```python
from build123d import *

# Parameters (mm, degrees)
SKETCH_2_W                   = 62
SKETCH_2_H                   = 45
EXTRUDE_3_DEPTH              = 8
SKETCH_3_W                   = 3.004963504
SKETCH_3_H                   = 5
CUT_EXTRUDE_1_DEPTH          = 58.648048048
EXTRUDE_4_DEPTH              = 3
SKETCH_6_W                   = 3
SKETCH_6_H                   = 5
EXTRUDE_5_DEPTH              = 2
SKETCH_7_W                   = 3
SKETCH_7_H                   = 5
EXTRUDE_6_DEPTH              = 2
SKETCH_8_W                   = 49.990072992
SKETCH_8_H                   = 5
EXTRUDE_7_DEPTH              = 2
SKETCH_9_W                   = 3
SKETCH_9_H                   = 5
CUT_EXTRUDE_2_DEPTH          = 66.65020057
SKETCH_10_W                  = 3
SKETCH_10_H                  = 5
CUT_EXTRUDE_4_DEPTH          = 66.65020057
SKETCH_11_W                  = 49.990072992
SKETCH_11_H                  = 5
EXTRUDE_8_DEPTH              = 17
SKETCH_12_W                  = 49.990072992
SKETCH_12_H                  = 3
EXTRUDE_9_DEPTH              = 25
EXTRUDE_START                = 3.72
SKETCH_16_W                  = 49.990072992
SKETCH_16_H                  = 25
EXTRUDE_10_DEPTH             = 3
SKETCH_17_W                  = 49.990072992
SKETCH_17_H                  = 25
CUT_EXTRUDE_5_DEPTH          = 81.043408441
SKETCH_18_W                  = 84
SKETCH_18_H                  = 3
EXTRUDE_11_DEPTH             = 20
HOLE_WIZARD_M3_2_D           = 2.5
HOLE_WIZARD_M3_2_CSINK_D     = 3.05
HOLE_WIZARD_M3_2_CSINK_ANGLE = 90


with BuildPart() as part:
    # 草图2 → 凸台-拉伸3 (new body)
    with BuildSketch(Plane.XY):
        with Locations((-4.132569558, -3.93531014)):
            Rectangle(SKETCH_2_W, SKETCH_2_H)
    extrude(amount=EXTRUDE_3_DEPTH)

    # 草图3 → 切除-拉伸1 (cut, through all)
    with BuildSketch(Plane.XZ.offset(26.43531014)):
        with Locations((-30.630087806, 5.5)):
            Rectangle(SKETCH_3_W, SKETCH_3_H)
        with Locations((22.36494869, 5.5)):
            Rectangle(SKETCH_3_W, SKETCH_3_H)
    extrude(amount=-CUT_EXTRUDE_1_DEPTH, mode=Mode.SUBTRACT)

    # 草图5 → 凸台-拉伸4 (add)
    with BuildSketch(Plane(origin=(0, 0, 0), x_dir=(-1, 0, 0), z_dir=(0, 0, -1))):
        Polygon((-38.867430442, -45.43531014), (-38.867430442, 18.56468986), (45.132569558, 18.56468986), (45.132569558, -45.43531014), (3.132569558, -45.43531014), align=None)
    extrude(amount=-EXTRUDE_4_DEPTH)

    # 草图6 → 凸台-拉伸5 (add)
    with BuildSketch(Plane.XZ.offset(26.43531014)):
        with Locations((-33.632569558, 5.5)):
            Rectangle(SKETCH_6_W, SKETCH_6_H)
    extrude(amount=EXTRUDE_5_DEPTH)

    # 草图7 → 凸台-拉伸6 (add)
    with BuildSketch(Plane.XZ.offset(26.43531014)):
        with Locations((25.367430442, 5.5)):
            Rectangle(SKETCH_7_W, SKETCH_7_H)
    extrude(amount=EXTRUDE_6_DEPTH)

    # 草图8 → 凸台-拉伸7 (add)
    with BuildSketch(Plane.XZ.offset(26.43531014)):
        with Locations((-4.132569558, 5.5)):
            Rectangle(SKETCH_8_W, SKETCH_8_H)
    extrude(amount=EXTRUDE_7_DEPTH)

    # 草图9 → 切除-拉伸2 (cut, through all)
    with BuildSketch(Plane.XZ.offset(28.43531014)):
        with Locations((-33.632569558, 5.5)):
            Rectangle(SKETCH_9_W, SKETCH_9_H)
    extrude(amount=-CUT_EXTRUDE_2_DEPTH, mode=Mode.SUBTRACT)

    # 草图10 → 切除-拉伸4 (cut, through all)
    with BuildSketch(Plane.XZ.offset(28.43531014)):
        with Locations((25.367430442, 5.5)):
            Rectangle(SKETCH_10_W, SKETCH_10_H)
    extrude(amount=-CUT_EXTRUDE_4_DEPTH, mode=Mode.SUBTRACT)

    # 草图11 → 凸台-拉伸8 (add)
    with BuildSketch(Plane.XZ.offset(28.43531014)):
        with Locations((-4.132569558, 5.5)):
            Rectangle(SKETCH_11_W, SKETCH_11_H)
    extrude(amount=EXTRUDE_8_DEPTH)

    # 草图12 → 凸台-拉伸9 (add)
    with BuildSketch(Plane.XY.offset(8)):
        with Locations((-4.132569558, -43.93531014)):
            Rectangle(SKETCH_12_W, SKETCH_12_H)
    extrude(amount=EXTRUDE_9_DEPTH)

    # 草图16 → 凸台-拉伸10 (add)
    with BuildSketch(Plane(origin=(0, -42.43531014, 0), x_dir=(1, 0, 0), z_dir=(0, 1, 0)).offset(EXTRUDE_START)):
        with Locations((-4.132569558, -20.5)):
            Rectangle(SKETCH_16_W, SKETCH_16_H)
    extrude(amount=EXTRUDE_10_DEPTH)

    # 草图17 → 切除-拉伸5 (cut, through all)
    with BuildSketch(Plane.XZ.offset(38.71531014)):
        with Locations((-4.132569558, 20.5)):
            Rectangle(SKETCH_17_W, SKETCH_17_H)
    extrude(amount=CUT_EXTRUDE_5_DEPTH, mode=Mode.SUBTRACT)

    # 草图18 → 凸台-拉伸11 (add)
    with BuildSketch(Plane.XZ.offset(45.43531014)):
        with Locations((-3.132569558, 1.5)):
            Rectangle(SKETCH_18_W, SKETCH_18_H)
    extrude(amount=EXTRUDE_11_DEPTH)

    # M3 螺纹孔2 (through all)
    with Locations(Plane.XY.offset(3)):
        with Locations((-43.132569558, -3.43531014), (36.867430442, -3.43531014), (36.867430442, -63.43531014), (-43.132569558, -63.43531014)):
            CounterSinkHole(HOLE_WIZARD_M3_2_D / 2, HOLE_WIZARD_M3_2_CSINK_D / 2, counter_sink_angle=HOLE_WIZARD_M3_2_CSINK_ANGLE)


solid = part.part
```
The listing builds one solid part. Answer for the finished solid, in the listing's coordinates (mm). A direction names the side the tool comes from. Give positions to 0.01 mm unless a question says otherwise; leave off trailing zeros. Write each loop counter-clockwise with the first axis right and the second up, starting at its lowest first coordinate (ties: lowest second). Pieces come first, ordered by that corner, then holes. Notation, with made-up numbers: (16.25, 86) -> (41.25, 86) arc R26 ccw to (41.25, 106) -> close; hole circle Ø11 at (77, 87). An arc over 180 degrees is marked (long way). Use one line per item in the form item = value.
1) A tool of negligible diameter and unlimited length cuts with its end or side. For faces 1 (the flat face through (-4, -35.715, 20)), 2 (the flat face through (-29.128, -18, 7)), 3 (the cylindrical face through (38.116, -3.38, 1.343)), 4 (the flat face through (-4, -42, 8)), 5 (the flat face through (-4, -23, 0)), from which of +Z, -Z, +X, -X, +Y, -Y can it reach the whole face along a straight path? Write none if from no direction.
Result:
face_1 = +Z, +X, -X, +Y
face_2 = +Z, -X, +Y, -Y
face_3 = +Z, -Z
face_4 = +Z, +X, -X, -Y
face_5 = -Z, +X, -X, +Y, -Y
2) Section D-D on y = -52.5 is taken. Write down the section's boundary in (x, z), plus the area to 3 significant figures.
Result:
outline = (-45.13, 0) -> (38.87, 0) -> (38.87, 3) -> (-45.13, 3) -> close
area = 252 mm²
3) Straight lines are drawn through the part: probe 1 along Z at (x, y) = (-33, -15); probe 2 along Y at (x, z) = (13, 10.5); probe 3 along Z at (x, y) = (20, 4). For each, find the intervals that lie inside material, in ascending order.
Result:
probe_1 = 0 to 3
probe_2 = -38.72 to -35.72
probe_3 = 0 to 8
4) Each of these flat-tipped pins is pushed along its axis until it touches: P1, Ø25, axis at x = -15, y = 0.5, coming from the +Z side; P2, Ø8, axis at x = 16.5, z = 29, coming from the -Y side; P3, Ø5, axis at x = 6, z = 27, coming from the +Y side. Where does it stop, or does it pass through?
Result:
P1 = 8
P2 = -38.72
P3 = -35.72
5) For a pull along Y with two mould halves and no side action, classify faces 6 (the cylindrical face through (-42.141, -4.196, 1.343)), 7 (the flat face through (-3, 18.565, 3)), 8 (the flat face through (-4, -38.715, 20)), 9 (the cylindrical face through (37.03, -62.196, 1.343)) as +Y half, -Y half, draft (parallel to the pull), parting line (faces both ways), or undercut.
Result:
face_6 = undercut
face_7 = +Y half
face_8 = -Y half
face_9 = undercut
6) Section A-A on y = -6 is taken. Write down the section's boundary in (x, z).
Result:
outline = (-45.13, 0) -> (38.87, 0) -> (38.87, 3) -> (20.86, 3) -> (20.86, 8) -> (-29.13, 8) -> (-29.13, 3) -> (-45.13, 3) -> close
7) Section B-B on x = -13 is taken. Write down the section's boundary in (y, z).
Result:
outline = (-65.44, 0) -> (18.56, 0) -> (18.56, 8) -> (-35.72, 8) -> (-35.72, 33) -> (-38.72, 33) -> (-38.72, 8) -> (-45.44, 8) -> (-45.44, 3) -> (-65.44, 3) -> close
8) Section C-C on z = 24.5 is taken. Write down the section's boundary in (x, y), plus the area to 3 significant figures.
Result:
outline = (-29.13, -38.72) -> (20.86, -38.72) -> (20.86, -35.72) -> (-29.13, -35.72) -> close
area = 150 mm²
